Autodesk Fusion 360 part; units mm, degrees
sketch "Skizze1" plane through (0, 0, 0) normal (0, 0, 1) x (1, 0, 0)
  line L0 (6.5, -4.75) -> (-6.5, -4.75)
  line L1 (-8.5, -2.75) -> (-8.5, 2.75)
  line L2 (-6.5, 4.75) -> (6.5, 4.75)
  line L3 (8.5, 2.75) -> (8.5, -2.75)
  line L4 (8.5, -4.75) -> (-8.5, 4.75) construction
  line L5 (-8.5, -4.75) -> (8.5, 4.75) construction
  arc A0 (-6.5, 4.75) -> (-8.5, 2.75) centre (-6.5, 2.75) ccw
  arc A1 (8.5, 2.75) -> (6.5, 4.75) centre (6.5, 2.75) ccw
  arc A2 (6.5, -4.75) -> (8.5, -2.75) centre (6.5, -2.75) ccw
  arc A3 (-8.5, -2.75) -> (-6.5, -4.75) centre (-6.5, -2.75) ccw
  line L6 (2.75, -2.25) -> (-2.75, -2.25)
  line L7 (-2.75, -2.25) -> (-2.75, 2.25)
  line L8 (-2.75, 2.25) -> (2.75, 2.25)
  line L9 (2.75, 2.25) -> (2.75, -2.25)
  line L10 (2.75, -2.25) -> (-2.75, 2.25) construction
  line L11 (-2.75, -2.25) -> (2.75, 2.25) construction
  line L12 (-2.75, 2.25) -> (-2.75, 4.75)
  line L13 (2.75, 2.25) -> (2.75, 4.75)
  arc A4 (-2.75, 2.25) -> (-2.75, 4.75) centre (-4.5, 3.5) ccw
  arc A5 (2.75, 4.75) -> (2.75, 2.25) centre (4.5, 3.5) ccw
  dimension "d487" = 17
  dimension "d488" = 9.5
  dimension "d489" = 2
  dimension "d491" = 5.5
  dimension "d492" = 4.5
  dimension "d501" = 9
extrude "Extrusion1" add sketch "Skizze1" along normal blind 1.5 contours L0 L1 L2 L3 A0 A1 A2 A3 L6 L7 L9 L12 L13 | L13 A5 | L12 A4
Could you check a few things on this model? Use its own coordinates, in mm. A direction names the side the tool comes from. Coordinates: 2 decimals unless noted, no trailing zeros. Write each loop counter-clockwise with the first axis right and the second up, starting at its lowest first coordinate (ties: lowest second). Pieces come first, ordered by that corner, then holes. Notation, with made-up numbers: M 85.25,-13.75 L 93.25,-13.75 A21 cw 93.25,5.25 Z; hole C 39.25,14 d4. An arc over 180 degrees is marked long. Answer as CSV lines item,"result". Start each with the question number.
1) I want a section at A-A, the plane y = 0.75. Please give me the cut outline in (x, z).
2) For faces 1 (the cylindrical face through (-2.35, 3.52, 0.74)), 2 (the cylindrical face through (-7.9, -4.18, 0.74)), which set-ups out of +Z, -Z, +X, -X, +Y, -Y let a thin tool reach every point of the face, with its end or its side?
3) We'd pull the mould along X, two halves only. Please class faces 3 (the cylindrical face through (7.9, 4.18, 0.74)), 4 (the flat face through (5, 4.75, 1)), 5 (the cylindrical face through (2.35, 3.48, 0.74)): +X half, -X half, draft (parallel to the pull), parting line (faces both ways), or undercut.
4) Please list where these lines run through material, in increasing order: line 1 (X direction, y = 1.5, z = 0.3); line 2 (Y direction, x = -1.75, z = 1.4); line 3 (X direction, y = 3, z = 0.8). Write a range as from..to.
5) I want a section at B-B, the plane z = 0.95. Please give me the cut outline in (x, y).
6) I want a section at C-C, the plane x = -2. Please give me the cut outline in (y, z).
7) I want a section at D-D, the plane y = 4. Please give me the cut outline in (x, z), and give its area (3 significant figures).
Data:
1,outline,"M -8.5,0 L -2.75,0 L -2.75,1.5 L -8.5,1.5 Z; M 2.75,0 L 8.5,0 L 8.5,1.5 L 2.75,1.5 Z"
2,face 1,"+Z, -Z"
2,face 2,"+Z, -Z, -X, -Y"
3,face 3,"+X half"
3,face 4,"draft"
3,face 5,"undercut"
4,line 1,"x = -8.5..-2.75, 2.75..8.5"
4,line 2,"y = -4.75..-2.25"
4,line 3,"x = -8.48..-2.41, 2.41..8.48"
5,outline,"M -8.5,-2.75 A2 ccw -6.5,-4.75 L 6.5,-4.75 A2 ccw 8.5,-2.75 L 8.5,2.75 A2 ccw 6.5,4.75 L 2.75,4.75 A2.15 ccw 2.75,2.25 L 2.75,-2.25 L -2.75,-2.25 L -2.75,2.25 A2.15 ccw -2.75,4.75 L -6.5,4.75 A2 ccw -8.5,2.75 Z"
6,outline,"M -4.75,0 L -2.25,0 L -2.25,1.5 L -4.75,1.5 Z"
7,outline,"M -8.06,0 L -2.41,0 L -2.41,1.5 L -8.06,1.5 Z; M 2.41,0 L 8.06,0 L 8.06,1.5 L 2.41,1.5 Z"
7,area,"17.0 mm^2"
